from build123d import *

# Parameters (mm, degrees)
F1_DEPTH = 16


with BuildPart() as f1:
    # F0 (on Front) → F1 (new body)
    with BuildSketch(Plane.XZ):
        with BuildLine():
            ThreePointArc((-11.633543, 2), (2.074661, 0), (-11.633543, -2))
            Line((-11.633543, -2), (-19.791408, -2))
            ThreePointArc((-19.791408, -2), (-19.212058, -4.57052), (-18.191838, -7))
            ThreePointArc((-18.191838, -7), (-6.752363, -14.888317), (6.255001, -10))
            ThreePointArc((6.255001, -10), (10.074661, 0), (6.255001, 10))
            ThreePointArc((6.255001, 10), (-6.752363, 14.888317), (-18.191838, 7))
            ThreePointArc((-18.191838, 7), (-19.212058, 4.57052), (-19.791408, 2))
            Line((-19.791408, 2), (-11.633543, 2))
        make_face()
        with BuildLine():
            ThreePointArc((-18.191838, -7), (-19.212058, -4.57052), (-19.791408, -2))
            Line((-19.791408, -2), (-29.925339, -2))
            Line((-29.925339, -2), (-29.925339, -7))
            Line((-29.925339, -7), (-18.191838, -7))
        make_face()
        with BuildLine():
            Line((-29.925339, 2), (-19.791408, 2))
            ThreePointArc((-19.791408, 2), (-19.212058, 4.57052), (-18.191838, 7))
            Line((-18.191838, 7), (-29.925339, 7))
            Line((-29.925339, 7), (-29.925339, 2))
        make_face()
        with BuildLine():
            ThreePointArc((6.255001, 10), (10.074661, 0), (6.255001, -10))
            Line((6.255001, -10), (54.441411, -10))
            ThreePointArc((54.441411, -10), (49.074661, 0), (54.441411, 10))
            Line((54.441411, 10), (6.255001, 10))
        make_face()
        with BuildLine():
            ThreePointArc((54.441411, 10), (49.074661, 0), (54.441411, -10))
            ThreePointArc((54.441411, -10), (63.236498, -11.803663), (70.821455, -7))
            ThreePointArc((70.821455, -7), (72.149986, -4.619219), (72.906821, -2))
            Line((72.906821, -2), (64.538763, -2))
            ThreePointArc((64.538763, -2), (57.074661, 0), (64.538763, 2))
            Line((64.538763, 2), (72.906821, 2))
            ThreePointArc((72.906821, 2), (72.149986, 4.619219), (70.821455, 7))
            ThreePointArc((70.821455, 7), (63.236498, 11.803663), (54.441411, 10))
        make_face()
        with BuildLine():
            ThreePointArc((72.906821, -2), (72.149986, -4.619219), (70.821455, -7))
            Line((70.821455, -7), (81.074661, -7))
            Line((81.074661, -7), (81.074661, -2))
            Line((81.074661, -2), (72.906821, -2))
        make_face()
        with BuildLine():
            Line((81.074661, 7), (70.821455, 7))
            ThreePointArc((70.821455, 7), (72.149986, 4.619219), (72.906821, 2))
            Line((72.906821, 2), (81.074661, 2))
            Line((81.074661, 2), (81.074661, 7))
        make_face()
    extrude(amount=F1_DEPTH)


solid = f1.part
Verification items for the finished model (mm, model axes). A direction names the side the tool comes from. Coordinates: 2 decimals unless noted, no trailing zeros. Order: outer loops, then holes, each group sorted by start corner. A loop starts at its lowest first (then second) coordinate and runs counter-clockwise, first axis right, second up. Notation, with made-up numbers: M 35,25 L 84,25 A32 ccw 84,60 Z; hole C 58,82.25 d9. An arc over 180 degrees is marked long. Return JSON: item names as keys, results as strings.
1) Cross-section at A-A, the plane y = -13. Record the boundary of the cut face in (x, z) (3 decimals).
Answer list:
{"outline": "M -29.925,-7 L -18.192,-7 A15 ccw 6.255,-10 L 54.441,-10 A12 ccw 70.821,-7 L 81.075,-7 L 81.075,-2 L 64.539,-2 A4 cw long 64.539,2 L 81.075,2 L 81.075,7 L 70.821,7 A12 ccw 54.441,10 L 6.255,10 A15 ccw -18.192,7 L -29.925,7 L -29.925,2 L -11.634,2 A7 cw long -11.634,-2 L -29.925,-2 Z"}
2) Cross-section at C-C, the plane x = 49. Record the boundary of the cut face in (y, z), and give its area (3 significant figures).
Answer list:
{"outline": "M -16,-10 L 0,-10 L 0,10 L -16,10 Z", "area": "320 mm2"}
3) Release check for a two-part mould opening along Z. For faces 5 (the flat face through (73, -8, 2)), 6 (the flat face through (-24, -8, 7)), 7 (the flat face through (-29.925, -8, -4)), 8 (the cylindrical face through (57.077, -7.888, -0.147)) record: +Z half, -Z half, draft (parallel to the pull), parting line (faces both ways), or undercut.
Answer list:
{"face 5": "undercut", "face 6": "+Z half", "face 7": "draft", "face 8": "undercut"}
4) Gauge pin test, flat ends, axial feed: pin 1 (8 mm diameter, centred on x = 40.5, y = -6, fed in from -Z); pin 2 (5 mm diameter, centred on x = 69.5, y = -4.5, fed in from -Z); pin 3 (2 mm diameter, centred on y = -8, z = 11.5, fed in from -X). Record the tip position at first contact, or that the pin passes through.
Answer list:
{"pin 1": "z = -10", "pin 2": "z = -10.44", "pin 3": "x = -15.64"}
5) Cross-section at B-B, the plane z = 5. Record the boundary of the cut face in (x, y), and give its area (3 significant figures).
Answer list:
{"outline": "M -29.93,-16 L -9.82,-16 L -9.82,0 L -29.93,0 Z; M -0.03,-16 L 81.07,-16 L 81.07,0 L -0.03,0 Z", "area": "1,620 mm2"}
6) Cross-section at D-D, the plane z = 0. Record the boundary of the cut face in (x, y), and give its area (3 significant figures).
Answer list:
{"outline": "M 2.07,-16 L 57.07,-16 L 57.07,0 L 2.07,0 Z", "area": "880 mm2"}
7) Thickness scan on L1, parallel to Z at x = 61, y = -13; L2, parallel to Z at x = 45, y = -12; L3, parallel to X at y = -14.75, z = 11. Record the ranges inside material, lowest first. Write a range as [from, to].
Answer list:
{"L1": "[-12, -4], [4, 12]", "L2": "[-10, 10]", "L3": "[-15.12, 5.27], [56.28, 65.87]"}
8) Access from +Z, -Z, +X, -X, +Y, -Y to the whole of each face (thin tool, end or side, straight path). Record for faces 1 (the flat face through (76, -8, -7)), 2 (the flat face through (31, -8, 10)), 3 (the flat face through (-21, -8, -2)), 4 (the flat face through (30, -8, -10)).
Answer list:
{"face 1": "-Z, +X, +Y, -Y", "face 2": "+Z, +Y, -Y", "face 3": "-X, +Y, -Y", "face 4": "-Z, +Y, -Y"}
